Input: part model. Units: mm. Frame: model coordinates. A direction names the side the tool comes from. Round coordinates to 2 decimals unless told otherwise and drop trailing zeros. Order: outer loops, then holes, each group sorted by start corner. A loop starts at its lowest first (then second) coordinate and runs counter-clockwise, first axis right, second up.
Item 1: Mould query, pull axis Z, two halves, no side actions, for faces 1 (the cylindrical face through (198.479, 35.291, 11.114)), 2 (the conical face through (177.555, 3.398, -10.789)), 3 (the flat face through (178.032, 0, -2)), 4 (the flat face through (-225, -8, 1)). Classes: released by +Z, released by -Z, zero draft, split by the parting line, or undercut.
Item 2: Line query: L1, parallel to X at y = -17.5, z = -31; L2, parallel to X at y = -21.5, z = -11.5; L3, parallel to Z at x = -13, y = 0. Output: solid intervals per line, ascending.
Item 3: First-contact query: pin 1 (5 mm diameter, centred on y = -19.5, z = -19, fed in from -X); pin 2 (3 mm diameter, centred on y = -9.5, z = 23.5, fed in from +X); pin 3 (3 mm diameter, centred on x = -274.5, z = 0.5, fed in from +Y); pin 4 (16 mm diameter, centred on y = 1, z = 4, fed in from -X). Flat tips, straight axial feed; report the tip coordinate or a pass-through.
Item 4: Reachability of faces 5 (the cylindrical face through (-25.645, 35.291, 11.114)), 6 (the flat face through (181.032, 0, 2)) from +Z, -Z, +X, -X, +Y, -Y: full face, straight path, thin tool, end or side. Return the list, or none.
Item 5: Cut plane A-A on x = -197.5. Output: boundary loops of the cut face in (y, z).
```python
from build123d import *

# Parameters (mm, degrees)
SKETCH2_R           = 2
BOSS_EXTRUDE1_DEPTH = 20
SKETCH5_R           = 0.5
CUT_EXTRUDE1_DEPTH  = 10


with BuildPart() as part:
    # Sketch1 → Revolve1 (revolve)
    with BuildSketch(Plane.XY):
        Polygon((-225, 2), (-225, 37), (225, 37), (260, 2), (410, 2), (410, 0), (-125, 0), (-325, 0), (-325, 2), align=None)
    revolve(axis=Axis((-125, 0, 0), (1, 0, 0)))

    # Sketch2 → Boss-Extrude1 (add)
    with BuildSketch(Plane(origin=(0, 0, 0), x_dir=(1, 0, 0), z_dir=(0, 1, 0))):
        with Locations((-275, 0)):
            Circle(SKETCH2_R)
        with Locations((335, 0)):
            Circle(SKETCH2_R)
    extrude(amount=BOSS_EXTRUDE1_DEPTH)


with BuildPart() as body_2:
    # Sketch4 → Revolve2 (revolve)
    with BuildSketch(Plane(origin=(0, 0, 0), x_dir=(1, 0, 0), z_dir=(0, 1, 0))):
        Polygon((181.031907012, 0), (181.031907012, 10), (171.204710687, 37), (168.204710687, 37), (178.031907012, 10), (178.031907012, 0), align=None)
    revolve(axis=Axis((178.031907012, 0, 0), (1, 0, 0)))

    # Sketch5 → Cut-Extrude1 (cut)
    with BuildSketch(Plane.ZY.offset(-178.031907012)):
        Circle(SKETCH5_R)
    extrude(amount=-CUT_EXTRUDE1_DEPTH, mode=Mode.SUBTRACT)


with BuildPart() as part_1:
    add(part.part)

    # Combine1: cut body 2
    add(body_2.part, mode=Mode.SUBTRACT)


solid = part_1.part
```
From the geometry:
1. face 1: split by the parting line
1. face 2: undercut
1. face 3: undercut
1. face 4: zero draft
2. L1: x = -225 to 168.71, 171.71 to 226.4
2. L2: x = -225 to 172.8, 175.8 to 237.62
2. L3: z = -37 to 37
3. pin 1: stops at x = -225
3. pin 2: stops at x = 238.15
3. pin 3: stops at y = 20
3. pin 4: stops at x = -325
4. face 5: +X, -X
4. face 6: none
5. outline: circle Ø74 at (0, 0)
